```python
from build123d import *

# Parameters (mm, degrees)
SKETCH1_W           = 77
SKETCH1_H           = 12
BOSS_EXTRUDE1_DEPTH = 10
SKETCH2_R           = 1.25
CUT_EXTRUDE1_DEPTH  = 12
SKETCH3_W           = 77
SKETCH3_H           = 20
BOSS_EXTRUDE2_DEPTH = 5


with BuildPart() as part:
    # Sketch1 → Boss-Extrude1 (new body)
    with BuildSketch(Plane.XY):
        with Locations((38.5, 6)):
            Rectangle(SKETCH1_W, SKETCH1_H)
    extrude(amount=BOSS_EXTRUDE1_DEPTH)

    # Sketch2 → Cut-Extrude1 (cut)
    with BuildSketch(Plane(origin=(77, 0, 0), x_dir=(0, 0, -1), z_dir=(1, 0, 0))):
        with Locations((-5, 3)):
            Circle(SKETCH2_R)
        with Locations((-5, 9)):
            Circle(SKETCH2_R)
    cut_extrude1 = extrude(amount=-CUT_EXTRUDE1_DEPTH, mode=Mode.SUBTRACT)

    # Mirror1: Cut-Extrude1 across plane
    add(cut_extrude1.mirror(Plane.ZY.offset(-38.5)), mode=Mode.SUBTRACT)

    # Sketch3 → Boss-Extrude2 (add)
    with BuildSketch(Plane(origin=(0, 12, 0), x_dir=(1, 0, 0), z_dir=(0, 1, 0))):
        with Locations((38.5, -10)):
            Rectangle(SKETCH3_W, SKETCH3_H)
    boss_extrude2 = extrude(amount=BOSS_EXTRUDE2_DEPTH)

    # Mirror2: Boss-Extrude2 across plane
    add(boss_extrude2.mirror(Plane(origin=(0, 6, 0), x_dir=(0, 0, 1), z_dir=(0, -1, 0))))


solid = part.part
```
Build history of the part. All positions in model axes, mm. A direction names the side the tool comes from. Coordinates: 2 decimals unless noted, no trailing zeros. Order: outer loops, then holes, each group sorted by start corner. A loop starts at its lowest first (then second) coordinate and runs counter-clockwise, first axis right, second up.
Item 1: Drill centre lines: L1, parallel to Y at x = 71.75, z = 5; L2, parallel to Y at x = 39, z = 10.5; L3, parallel to Z at x = 28.5, y = 5.25. Where is each one in solid material? Low to high.
Filled in:
L1: y = -5 to 1.75, 4.25 to 7.75, 10.25 to 17
L2: y = -5 to 0, 12 to 17
L3: z = 0 to 10
Item 2: Drop flat-ended pins along their axis: pin 1 Ø2 at (y, z) = (3, 5) entering from +X; pin 2 Ø3.5 at (x, y) = (34, 8) entering from +Z; pin 3 Ø0.8 at (y, z) = (9.5, 5) entering from -X. Give the stop position or say it passes through.
Filled in:
pin 1: stops at x = 65
pin 2: stops at z = 10
pin 3: stops at x = 12
Item 3: Saw through at B-B on x = 29.5. List the corners of the cut face in (y, z), then the cut area to 3 significant figures.
Filled in:
outline: (-5, 0) - (17, 0) - (17, 20) - (12, 20) - (12, 10) - (0, 10) - (0, 20) - (-5, 20) - close
area: 320 mm2
Item 4: Tool access for faces 1 (the flat face through (77, 6, 8)), 2 (the cylindrical face through (71.084, 3.845, 5.921)), 3 (the flat face through (12, 9, 5)), 4 (the flat face through (38, 0, 15)): list every direction of +Z, -Z, +X, -X, +Y, -Y with a clear straight run to the whole face (end or side of a thin tool).
Filled in:
face 1: +Z, -Z, +X, +Y, -Y
face 2: +X
face 3: -X
face 4: +Z, +X, -X
Item 5: Saw through at D-D on z = 5. List the corners of the cut face in (x, y).
Filled in:
outline: (0, -5) - (77, -5) - (77, 1.75) - (65, 1.75) - (65, 4.25) - (77, 4.25) - (77, 7.75) - (65, 7.75) - (65, 10.25) - (77, 10.25) - (77, 17) - (0, 17) - (0, 10.25) - (12, 10.25) - (12, 7.75) - (0, 7.75) - (0, 4.25) - (12, 4.25) - (12, 1.75) - (0, 1.75) - close
Item 6: Saw through at A-A on z = 16.5. List the corners of the cut face in (x, y), then the cut area to 3 significant figures.
Filled in:
outline: (0, -5) - (77, -5) - (77, 0) - (0, 0) - close; (0, 12) - (77, 12) - (77, 17) - (0, 17) - close
area: 770 mm2
Item 7: Saw through at C-C on y = 3. List the corners of the cut face in (x, z).
Filled in:
outline: (0, 0) - (77, 0) - (77, 3.75) - (65, 3.75) - (65, 6.25) - (77, 6.25) - (77, 10) - (0, 10) - (0, 6.25) - (12, 6.25) - (12, 3.75) - (0, 3.75) - close
Item 8: Mould opens along Y. For faces 5 (the flat face through (38, -5, 10)), 6 (the flat face through (38, 14, 20)), 7 (the cylindrical face through (5.916, 3.845, 5.921)) say: released by +Y, released by -Y, zero draft, split by the parting line, or undercut.
Filled in:
face 5: released by -Y
face 6: zero draft
face 7: undercut
